Source: CAD feature listing. Evaluate the final solid. Frame: model axes, mm. Face numbers are marked on the shaded views. A direction names the side the tool comes from. Give positions to 0.01 mm unless a question says otherwise; leave off trailing zeros. Write each loop counter-clockwise with the first axis right and the second up, starting at its lowest first coordinate (ties: lowest second). Pieces come first, ordered by that corner, then holes. Notation, with made-up numbers: (80, 58.25) -> (134, 58.25) arc R21 cw to (134, 83.25) -> close; hole circle Ø5 at (42.25, 12.5). An arc over 180 degrees is marked (long way). Write item = value, one per line.
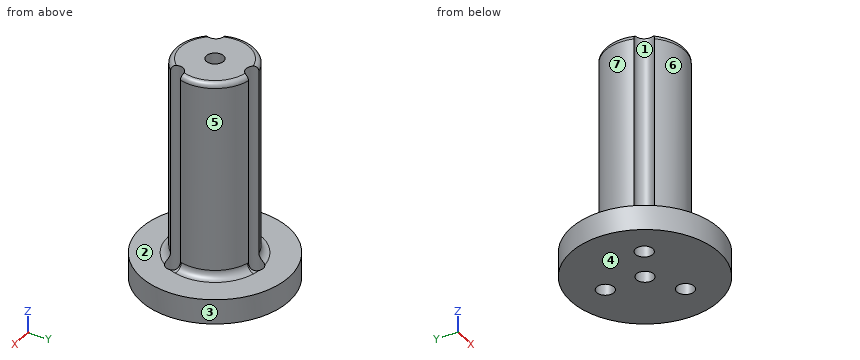
from build123d import *

# Parameters (mm, degrees)
SKETCH_1_R          = 15
EXTRUDE_1_DEPTH     = 5
SKETCH_2_R          = 8
EXTRUDE_2_DEPTH     = 40
SKETCH_3_R          = 1.75
CUT_EXTRUDE_1_DEPTH = 49
FILLET_1_R          = 1.5
FILLET_2_R          = 1


with BuildPart() as part:
    # 草图1 → 凸台-拉伸1 (new body)
    with BuildSketch(Plane.XY):
        Circle(SKETCH_1_R)
    extrude(amount=EXTRUDE_1_DEPTH)

    # 草图2 → 凸台-拉伸2 (add)
    with BuildSketch(Plane.XY.offset(5)):
        Circle(SKETCH_2_R)
    extrude(amount=EXTRUDE_2_DEPTH)

    # 草图3 → 切除-拉伸1 (cut)
    with BuildSketch(Plane(origin=(0, 0, 0), x_dir=(-1, 0, 0), z_dir=(0, 0, -1))):
        with Locations((0, 8)):
            Circle(SKETCH_3_R)
        Circle(SKETCH_3_R)
        with Locations((6.92820323, -4)):
            Circle(SKETCH_3_R)
        with Locations((-6.92820323, -4)):
            Circle(SKETCH_3_R)
    extrude(amount=-CUT_EXTRUDE_1_DEPTH, mode=Mode.SUBTRACT)

    # 圆角1
    # the kernel refuses this fillet: 1.5 mm, written as the material it adds along each edge
    with BuildSketch(Plane(origin=(0, 0, 5), x_dir=(0.24718186036796463, 0.968969105753652, 0), z_dir=(0.968969105753652, -0.24718186036796463, 0))) as fillet_1_piece_1_section:
        with BuildLine():
            CenterArc((8 + FILLET_1_R, FILLET_1_R), FILLET_1_R, 180, 90)
            Line((8, FILLET_1_R), (8, 0))
            Line((8, 0), (8 + FILLET_1_R, 0))
        make_face()
    fillet_1_piece_1 = revolve(axis=Axis((0, 0, 5), (0, 0, 1)), revolution_arc=148.621623282, mode=Mode.PRIVATE)
    fillet_1_piece_1 = fillet_1_piece_1 - Plane(origin=(-6.92820323, -4, 5.2649635), x_dir=(-1, 0, 0), z_dir=(0, 0, -1)) * Cylinder(1.75, 39, mode=Mode.PRIVATE)
    fillet_1_piece_1 = fillet_1_piece_1 - Plane(origin=(0, 8, 5.2649635), x_dir=(-1, 0, 0), z_dir=(0, 0, -1)) * Cylinder(1.75, 39, mode=Mode.PRIVATE)
    add(fillet_1_piece_1)
    with BuildSketch(Plane(origin=(0, 0, 5), x_dir=(-0.9627427912489371, -0.27041878244346385, 0), z_dir=(-0.27041878244346385, 0.9627427912489371, 0))) as fillet_1_piece_2_section:
        with BuildLine():
            CenterArc((8 + FILLET_1_R, FILLET_1_R), FILLET_1_R, 180, 90)
            Line((8, FILLET_1_R), (8, 0))
            Line((8, 0), (8 + FILLET_1_R, 0))
        make_face()
    fillet_1_piece_2 = revolve(axis=Axis((0, 0, 5), (0, 0, 1)), revolution_arc=148.621623282, mode=Mode.PRIVATE)
    fillet_1_piece_2 = fillet_1_piece_2 - Plane(origin=(6.92820323, -4, 5.2649635), x_dir=(-1, 0, 0), z_dir=(0, 0, -1)) * Cylinder(1.75, 39, mode=Mode.PRIVATE)
    fillet_1_piece_2 = fillet_1_piece_2 - Plane(origin=(-6.92820323, -4, 5.2649635), x_dir=(-1, 0, 0), z_dir=(0, 0, -1)) * Cylinder(1.75, 39, mode=Mode.PRIVATE)
    add(fillet_1_piece_2)
    with BuildSketch(Plane(origin=(0, 0, 5), x_dir=(-0.24718186036796455, 0.968969105753652, 0), z_dir=(-0.968969105753652, -0.24718186036796455, 0))) as fillet_1_piece_3_section:
        with BuildLine():
            CenterArc((8 + FILLET_1_R, -FILLET_1_R), FILLET_1_R, 90, 90)
            Line((8, -FILLET_1_R), (8, 0))
            Line((8, 0), (8 + FILLET_1_R, 0))
        make_face()
    fillet_1_piece_3 = revolve(axis=Axis((0, 0, 5), (0, 0, -1)), revolution_arc=148.621623282, mode=Mode.PRIVATE)
    fillet_1_piece_3 = fillet_1_piece_3 - Plane(origin=(6.92820323, -4, 5.264963506), x_dir=(-1, 0, 0), z_dir=(0, 0, -1)) * Cylinder(1.75, 39, mode=Mode.PRIVATE)
    fillet_1_piece_3 = fillet_1_piece_3 - Plane(origin=(0, 8, 5.264963506), x_dir=(-1, 0, 0), z_dir=(0, 0, -1)) * Cylinder(1.75, 39, mode=Mode.PRIVATE)
    add(fillet_1_piece_3)

    # 圆角2
    fillet_2_edges = [part.edges().sort_by_distance(p)[0] for p in [
        (-6.92820323, 4, 45),
        (0, -8, 45),
        (6.92820323, 4, 45),
    ]]
    fillet(fillet_2_edges, radius=FILLET_2_R)


solid = part.part
1) Cut plane C-C (z = 29). Return the cut outline in (x, y).
Computed:
outline = (-7.63, -2.4) arc R1.75 cw to (-5.89, -5.41) arc R8 ccw to (5.89, -5.41) arc R1.75 cw to (7.63, -2.4) arc R8 ccw to (1.74, 7.81) arc R1.75 cw to (-1.74, 7.81) arc R8 ccw to start; hole circle Ø3.5 at (0, 0)
2) Material intervals for L1, parallel to Y at x = 0, z = 34.5; L2, parallel to X at y = -4, z = 31.5; L3, parallel to Z at x = 9.25, y = -6.75, sorted ascending.
Computed:
L1 = -8 to -1.75, 1.75 to 6.25
L2 = -5.18 to 5.18
L3 = 0 to 5
3) Cut plane D-D (x = 10). Return the cut outline in (y, z), then the cut area to 3 significant figures.
Computed:
outline = (-11.18, 0) -> (11.18, 0) -> (11.18, 5) -> (-11.18, 5) -> close
area = 112 mm²
4) Cut plane B-B (x = 0). Return the cut outline in (y, z), then the cut area to 3 significant figures.
Computed:
outline = (-15, 0) -> (-1.75, 0) -> (-1.75, 45) -> (-7, 45) arc R1 ccw to (-8, 44) -> (-8, 6.5) arc R1.5 cw to (-9.5, 5) -> (-15, 5) -> close; (1.75, 0) -> (6.25, 0) -> (6.25, 45) -> (1.75, 45) -> close; (9.75, 0) -> (15, 0) -> (15, 5) -> (9.75, 5) -> close
area = 545 mm²
5) Access query for the marked faces 4, 5, 6 and 7. Directions: +Z, -Z, +X, -X, +Y, -Y. A direction counts if a zero-diameter tool reaches every point of the face in a straight line with its end or side. Return the directions, or none.
Computed:
face_4 = -Z, +X, -X, +Y, -Y
face_5 = +Z, +X
face_6 = +Z, -Y
face_7 = +Z, -X
6) Draft query along Y for the marked faces 1, 2 and 3. Return one class per face: pulls with the +Y half, pulls with the -Y half, needs draft (parallel to the pull), parting line crosses it, or undercut.
Computed:
face_1 = undercut
face_2 = needs draft
face_3 = parting line crosses it
7) Cut plane A-A (y = 0). Return the cut outline in (x, z), then the cut area to 3 significant figures.
Computed:
outline = (-15, 0) -> (-1.75, 0) -> (-1.75, 45) -> (-7, 45) arc R1 ccw to (-8, 44) -> (-8, 6.5) arc R1.5 cw to (-9.5, 5) -> (-15, 5) -> close; (1.75, 0) -> (15, 0) -> (15, 5) -> (9.5, 5) arc R1.5 cw to (8, 6.5) -> (8, 44) arc R1 ccw to (7, 45) -> (1.75, 45) -> close
area = 633 mm²
8) Contact query for flat-ended pins moving along their axis: pin 1 (4.5 mm diameter, centred on x = 0, y = 8, fed in from +Z); pin 2 (6 mm diameter, centred on x = 0, z = 12, fed in from +Y); pin 3 (8 mm diameter, centred on y = -1, z = 20, fed in from -X); pin 4 (6 mm diameter, centred on x = -9.5, z = 15.5, fed in from -Y). Output: stop coordinate, or through.
Computed:
pin_1 = 45
pin_2 = 7.81
pin_3 = -8
pin_4 = -2.4
